from build123d import *

# Parameters (mm, degrees)
SKETCH1_W                       = 120
SKETCH1_H                       = 50
BOSS_EXTRUDE1_DEPTH             = 6
SKETCH2_W                       = 50
SKETCH2_H                       = 10
BOSS_EXTRUDE2_DEPTH             = 12
SKETCH3_R                       = 1.7
CUT_EXTRUDE1_DEPTH              = 19
SKETCH5_W                       = 10
SKETCH5_H                       = 12
CUT_EXTRUDE2_DEPTH              = 37
CBORE_FOR_M3_SBHCS2_D           = 3.4
CBORE_FOR_M3_SBHCS2_DEPTH       = 3.15
CBORE_FOR_M3_SBHCS2_CBORE_D     = 6.7
CBORE_FOR_M3_SBHCS2_CBORE_DEPTH = 1.65
CBORE_FOR_M3_SBHCS2_TIP         = 1.021463052
SKETCH6_R                       = 1.7
CUT_EXTRUDE3_DEPTH              = 6
CBORE_FOR_M3_SBHCS3_D           = 3.4
CBORE_FOR_M3_SBHCS3_DEPTH       = 3.15
CBORE_FOR_M3_SBHCS3_CBORE_D     = 6.7
CBORE_FOR_M3_SBHCS3_CBORE_DEPTH = 1.65
CBORE_FOR_M3_SBHCS3_TIP         = 1.021463052
SKETCH9_R                       = 3.2
CUT_EXTRUDE4_DEPTH              = 7
SKETCH10_W                      = 22
SKETCH10_H                      = 42
CUT_EXTRUDE5_DEPTH              = 6.5
SKETCH11_W                      = 22
SKETCH11_H                      = 7
SKETCH11_R                      = 2.2
BOSS_EXTRUDE4_DEPTH             = 2
CUT_EXTRUDE6_START              = -6
SKETCH12_R                      = 2.2
CUT_EXTRUDE6_DEPTH              = 6


with BuildPart() as part:
    # Sketch1 → Boss-Extrude1 (new body)
    with BuildSketch(Plane(origin=(0, 0, 0), x_dir=(0, 1, 0), z_dir=(0, 0, 1))):
        Rectangle(SKETCH1_W, SKETCH1_H)
    extrude(amount=BOSS_EXTRUDE1_DEPTH)

    # Sketch2 → Boss-Extrude2 (add)
    with BuildSketch(Plane(origin=(0, 0, 0), x_dir=(1, 0, 0), z_dir=(0, 0, -1))):
        with Locations((0, 55)):
            Rectangle(SKETCH2_W, SKETCH2_H)
        with Locations((0, -55)):
            Rectangle(SKETCH2_W, SKETCH2_H)
    extrude(amount=BOSS_EXTRUDE2_DEPTH)

    # Sketch3 → Cut-Extrude1 (cut)
    with BuildSketch(Plane.XY.offset(6)):
        with Locations((-19, -55)):
            Circle(SKETCH3_R)
        with Locations(Location((-19, 55, 0), (0, 0, 180))):
            Circle(SKETCH3_R)
    extrude(amount=-CUT_EXTRUDE1_DEPTH, mode=Mode.SUBTRACT)

    # Sketch5 → Cut-Extrude2 (cut)
    with BuildSketch(Plane.YZ.offset(25)):
        with Locations((-55, -6)):
            Rectangle(SKETCH5_W, SKETCH5_H)
        with Locations((55, -6)):
            Rectangle(SKETCH5_W, SKETCH5_H)
    extrude(amount=-CUT_EXTRUDE2_DEPTH, mode=Mode.SUBTRACT)

    # CBORE for M3 SBHCS2
    with Locations(Plane(origin=(-19, 55, 6), x_dir=(1, 0, 0), z_dir=(0, 0, 1))):
        with Locations((0, 0), (0, -110)):
            CounterBoreHole(CBORE_FOR_M3_SBHCS2_D / 2, CBORE_FOR_M3_SBHCS2_CBORE_D / 2, CBORE_FOR_M3_SBHCS2_CBORE_DEPTH, depth=CBORE_FOR_M3_SBHCS2_DEPTH)
            with Locations((0, 0, -(CBORE_FOR_M3_SBHCS2_DEPTH + CBORE_FOR_M3_SBHCS2_TIP / 2))):  # 118° drill point
                Cone(0, CBORE_FOR_M3_SBHCS2_D / 2, CBORE_FOR_M3_SBHCS2_TIP, mode=Mode.SUBTRACT)

    # Sketch6 → Cut-Extrude3 (cut)
    with BuildSketch(Plane(origin=(0, 0, 0), x_dir=(1, 0, 0), z_dir=(0, 0, -1))):
        with Locations(Location((19, 4, 0), (0, 0, 180))):
            Circle(SKETCH6_R)
    extrude(amount=-CUT_EXTRUDE3_DEPTH, mode=Mode.SUBTRACT)

    # CBORE for M3 SBHCS3
    with Locations(Plane(origin=(19, -4, 6), x_dir=(1, 0, 0), z_dir=(0, 0, 1))):
        with Locations((0, 0)):
            CounterBoreHole(CBORE_FOR_M3_SBHCS3_D / 2, CBORE_FOR_M3_SBHCS3_CBORE_D / 2, CBORE_FOR_M3_SBHCS3_CBORE_DEPTH, depth=CBORE_FOR_M3_SBHCS3_DEPTH)
            with Locations((0, 0, -(CBORE_FOR_M3_SBHCS3_DEPTH + CBORE_FOR_M3_SBHCS3_TIP / 2))):  # 118° drill point
                Cone(0, CBORE_FOR_M3_SBHCS3_D / 2, CBORE_FOR_M3_SBHCS3_TIP, mode=Mode.SUBTRACT)

    # Sketch9 → Cut-Extrude4 (cut)
    with BuildSketch(Plane.XY.offset(6)):
        with Locations((0.12, -22.03)):
            Circle(SKETCH9_R)
    extrude(amount=-CUT_EXTRUDE4_DEPTH, mode=Mode.SUBTRACT)

    # Sketch10 → Cut-Extrude5 (cut)
    with BuildSketch(Plane.XY.offset(6)):
        with Locations((0.12, -12.03)):
            Rectangle(SKETCH10_W, SKETCH10_H)
    extrude(amount=-CUT_EXTRUDE5_DEPTH, mode=Mode.SUBTRACT)

    # Sketch11 → Boss-Extrude4 (add)
    # profile 1 of 2: a face of its own
    with BuildSketch(Plane.XY.offset(6)):
        with Locations((0.12, -36.53)):
            Rectangle(SKETCH11_W, SKETCH11_H)
        with Locations((-4.88, -36.53)):
            Circle(SKETCH11_R, mode=Mode.SUBTRACT)
        with Locations((5.12, -36.53)):
            Circle(SKETCH11_R, mode=Mode.SUBTRACT)
    # profile 2 of 2: a face of its own
    with BuildSketch(Plane.XY.offset(6)):
        with Locations((0.12, 12.47)):
            Rectangle(SKETCH11_W, SKETCH11_H)
        with Locations(Location((5.12, 12.47, 0), (0, 0, 180))):
            Circle(SKETCH11_R, mode=Mode.SUBTRACT)
        with Locations(Location((-4.88, 12.47, 0), (0, 0, 180))):
            Circle(SKETCH11_R, mode=Mode.SUBTRACT)
    extrude(amount=BOSS_EXTRUDE4_DEPTH)

    # Sketch12 → Cut-Extrude6 (cut)
    with BuildSketch(Plane.XY.offset(6).offset(CUT_EXTRUDE6_START)):
        with Locations((-4.88, -36.53)):
            Circle(SKETCH12_R)
        with Locations((5.12, -36.53)):
            Circle(SKETCH12_R)
        with Locations(Location((-4.88, 12.47, 0), (0, 0, 180))):
            Circle(SKETCH12_R)
        with Locations(Location((5.12, 12.47, 0), (0, 0, 180))):
            Circle(SKETCH12_R)
    extrude(amount=CUT_EXTRUDE6_DEPTH, mode=Mode.SUBTRACT)


solid = part.part
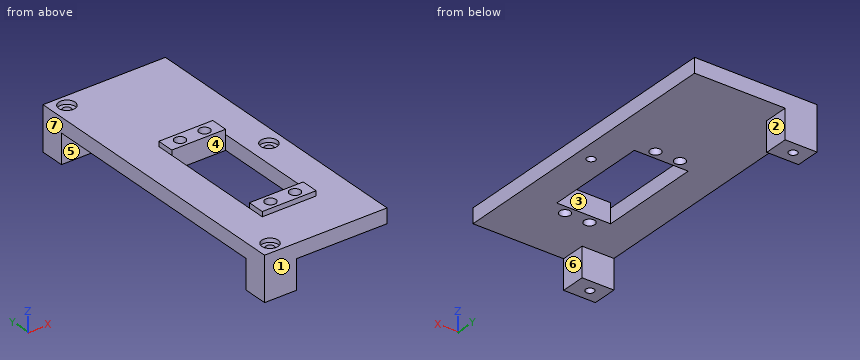
Geometry: final body of the model. Coordinates: model frame, mm. Face numbers are marked on the shaded views. A direction names the side the tool comes from. Round coordinates to 2 decimals unless told otherwise and drop trailing zeros. Loops run counter-clockwise (first coordinate to the right, second up) from the corner with the lowest first, then second, coordinate; pieces in that order, holes last.
Q1. Material intervals for L1, parallel to Y at x = -4.88, z = 3.5; L2, parallel to X at y = 12.47, z = 5; L3, parallel to Y at x = -19, z = 5.5, sorted ascending.
Q2. Pull-direction query (X, two-part tool) for the marked faces 1, 2, 3 and 4; classes: released by +X, released by -X, zero draft, split by the parting line, or undercut.
Q3. Section B-B on x = -4.88. Return loops of the section in (y, z), plus the area to 3 significant figures.
Q4. Section C-C on z = -6.75. Return loops of the section in (x, y), plus the area to 3 significant figures.
Q5. Pin query (flat end, axial travel): P1, Ø5, axis at y = 24.5, z = -3.5, coming from the -X side; P2, Ø8, axis at y = 53, z = -8, coming from the +X side; P3, Ø7.5, axis at x = -18.5, y = 54.5, coming from the +Z side; P4, Ø4.5, axis at x = -19, y = -55, coming from the +Z side. Return the tip coordinate at first contact, or that it passes through.
Q6. Section A-A on y = -16. Return loops of the section in (x, z), plus the area to 3 significant figures.
Q7. Access query for the marked faces 5, 6 and 7. Directions: +Z, -Z, +X, -X, +Y, -Y. A direction counts if a zero-diameter tool reaches every point of the face in a straight line with its end or side. Return the directions, or none.
Q8. Section D-D on x = -19. Return loops of the section in (y, z), plus the area to 3 significant figures.
Evaluation:
1. L1: y = -60 to -38.73, -34.33 to -33.03, 8.97 to 10.27, 14.67 to 60
1. L2: x = -25 to -7.08, -2.68 to 2.92, 7.32 to 25
1. L3: y = -60 to -58.35, -51.65 to 51.65, 58.35 to 60
2. face 1: zero draft
2. face 2: released by +X
2. face 3: undercut
2. face 4: undercut
3. outline: (-60, 0) - (-38.73, 0) - (-38.73, 8) - (-40.03, 8) - (-40.03, 6) - (-60, 6) - close; (-34.33, 0) - (-33.03, 0) - (-33.03, 8) - (-34.33, 8) - close; (8.97, 0) - (10.27, 0) - (10.27, 8) - (8.97, 8) - close; (14.67, 0) - (60, 0) - (60, 6) - (15.97, 6) - (15.97, 8) - (14.67, 8) - close
3. area: 426 mm2
4. outline: (-25, -60) - (-12, -60) - (-12, -50) - (-25, -50) - close; (-25, 50) - (-12, 50) - (-12, 60) - (-25, 60) - close; hole circle Ø3.4 at (-19, -55); hole circle Ø3.4 at (-19, 55)
4. area: 242 mm2
5. P1: passes through
5. P2: stops at x = -12
5. P3: stops at z = 6
5. P4: stops at z = 4.35
6. outline: (-25, 0) - (-10.88, 0) - (-10.88, 6) - (-25, 6) - close; (11.12, 0) - (25, 0) - (25, 6) - (11.12, 6) - close
6. area: 168 mm2
7. face 5: -Z, +X, -X
7. face 6: -Z, +X, +Y, -Y
7. face 7: +Z, -Z, -X, +Y, -Y
8. outline: (-60, -12) - (-56.7, -12) - (-56.7, 4.35) - (-58.35, 4.35) - (-58.35, 6) - (-60, 6) - close; (-53.3, -12) - (-50, -12) - (-50, 0) - (50, 0) - (50, -12) - (53.3, -12) - (53.3, 4.35) - (51.65, 4.35) - (51.65, 6) - (-51.65, 6) - (-51.65, 4.35) - (-53.3, 4.35) - close; (56.7, -12) - (60, -12) - (60, 6) - (58.35, 6) - (58.35, 4.35) - (56.7, 4.35) - close
8. area: 827 mm2
